from build123d import *

# Parameters (mm, degrees)
EXTRUDE_1_DEPTH       = 244
EXTRUDE_3_DEPTH       = 244
PATTERN_CURVE_1_DEPTH = 244
SKETCH_3_R            = 2.25
CUT_EXTRUDE_1_DEPTH   = 6
SKETCH_4_R            = 1.6
SKETCH_4_R_2          = 1.15
CUT_EXTRUDE_2_DEPTH   = 6


# Read off the part's stored shape, not the designer's step: the pattern curve step
with BuildPart() as part:
    # Sketch 1 → Extrude 1 (new body)
    with BuildSketch(Plane.XY):
        with BuildLine():
            Line((0, 40), (1.528979332, 40))
            ThreePointArc((1.528979332, 40), (2.225614441, 39.717425624), (2.528547087, 39.029399052))
            Line((2.528547087, 39.029399052), (3.5, 6))
            Line((3.5, 6), (118.5, 6))
            Line((118.5, 6), (119.471452913, 39.029399052))
            ThreePointArc((119.471452913, 39.029399052), (119.774385559, 39.717425624), (120.471020668, 40))
            Line((120.471020668, 40), (122, 40))
            Line((122, 40), (122, 0))
            Line((122, 0), (0, 0))
            Line((0, 0), (0, 40))
        make_face()
    extrude(amount=EXTRUDE_1_DEPTH)

    # Sketch 2 → Extrude 3 (add)
    with BuildSketch(Plane.XY.offset(244)):
        with BuildLine():
            Line((10.5, 39.5), (9.25, 6))
            Line((9.25, 6), (12.75, 6))
            Line((12.75, 6), (11.5, 39.5))
            ThreePointArc((11.5, 39.5), (11, 40), (10.5, 39.5))
        make_face()
    extrude(amount=-EXTRUDE_3_DEPTH)

    # Pattern Curve 1 outline → Pattern Curve 1 (add)
    with BuildSketch(Plane.XY):
        with BuildLine():
            ThreePointArc((21.5, 39.5), (21, 40), (20.5, 39.5))
            Line((20.5, 39.5), (19.25, 6))
            Line((19.25, 6), (22.75, 6))
            Line((22.75, 6), (21.5, 39.5))
        make_face()
        with BuildLine():
            Line((110.5, 39.5), (109.25, 6))
            Line((109.25, 6), (112.75, 6))
            Line((112.75, 6), (111.5, 39.5))
            ThreePointArc((111.5, 39.5), (111, 40), (110.5, 39.5))
        make_face()
        with BuildLine():
            Line((100.5, 39.5), (99.25, 6))
            Line((99.25, 6), (102.75, 6))
            Line((102.75, 6), (101.5, 39.5))
            ThreePointArc((101.5, 39.5), (101, 40), (100.5, 39.5))
        make_face()
        with BuildLine():
            Line((90.5, 39.5), (89.25, 6))
            Line((89.25, 6), (92.75, 6))
            Line((92.75, 6), (91.5, 39.5))
            ThreePointArc((91.5, 39.5), (91, 40), (90.5, 39.5))
        make_face()
        with BuildLine():
            Line((80.5, 39.5), (79.25, 6))
            Line((79.25, 6), (82.75, 6))
            Line((82.75, 6), (81.5, 39.5))
            ThreePointArc((81.5, 39.5), (81, 40), (80.5, 39.5))
        make_face()
        with BuildLine():
            Line((70.5, 39.5), (69.25, 6))
            Line((69.25, 6), (72.75, 6))
            Line((72.75, 6), (71.5, 39.5))
            ThreePointArc((71.5, 39.5), (71, 40), (70.5, 39.5))
        make_face()
        with BuildLine():
            Line((60.5, 39.5), (59.25, 6))
            Line((59.25, 6), (62.75, 6))
            Line((62.75, 6), (61.5, 39.5))
            ThreePointArc((61.5, 39.5), (61, 40), (60.5, 39.5))
        make_face()
        with BuildLine():
            Line((50.5, 39.5), (49.25, 6))
            Line((49.25, 6), (52.75, 6))
            Line((52.75, 6), (51.5, 39.5))
            ThreePointArc((51.5, 39.5), (51, 40), (50.5, 39.5))
        make_face()
        with BuildLine():
            Line((40.5, 39.5), (39.25, 6))
            Line((39.25, 6), (42.75, 6))
            Line((42.75, 6), (41.5, 39.5))
            ThreePointArc((41.5, 39.5), (41, 40), (40.5, 39.5))
        make_face()
        with BuildLine():
            Line((30.5, 39.5), (29.25, 6))
            Line((29.25, 6), (32.75, 6))
            Line((32.75, 6), (31.5, 39.5))
            ThreePointArc((31.5, 39.5), (31, 40), (30.5, 39.5))
        make_face()
    extrude(amount=PATTERN_CURVE_1_DEPTH)

    # Sketch 3 → Cut-Extrude 1 (cut)
    with BuildSketch(Plane.XZ):
        with Locations((26, 236)):
            Circle(SKETCH_3_R)
        with Locations((96, 236)):
            Circle(SKETCH_3_R)
        with Locations(Location((96, 8, 0), (0, 0, 180))):
            Circle(SKETCH_3_R)
        with Locations(Location((26, 8, 0), (0, 0, 180))):
            Circle(SKETCH_3_R)
    extrude(amount=-CUT_EXTRUDE_1_DEPTH, mode=Mode.SUBTRACT)

    # Sketch 4 → Cut-Extrude 2 (cut)
    with BuildSketch(Plane(origin=(133.240090243, 0, 310.149074448), x_dir=(-1, 0, 0), z_dir=(0, -1, 0))):
        with Locations((8.990090243, 225.549074448)):
            Circle(SKETCH_4_R)
        with Locations(Location((83.240090243, 178.149074448, 0), (0, 0, 180))):
            Circle(SKETCH_4_R_2)
        with Locations(Location((69.240090243, 163.149074448, 0), (0, 0, 180))):
            Circle(SKETCH_4_R)
        with Locations(Location((61.240090243, 283.149074448, 0), (0, 0, 180))):
            Circle(SKETCH_4_R)
        with Locations(Location((61.240090243, 178.149074448, 0), (0, 0, 180))):
            Circle(SKETCH_4_R)
        with Locations(Location((107.240090243, 178.149074448, 0), (0, 0, 180))):
            Circle(SKETCH_4_R_2)
    extrude(amount=-CUT_EXTRUDE_2_DEPTH, mode=Mode.SUBTRACT)


solid = part.part
Build history of the part. All positions in model axes, mm. A direction names the side the tool comes from. Coordinates: 2 decimals unless noted, no trailing zeros. Use CSV: the item, a comma, the result in double quotes. Start each with the question number.
Q1. 3-axis set-ups, long thin cutter, end or side, ignore diameter. For faces 3 (the flat face through (0, 20, 120)), 4 (the flat face through (46, 6, 120)): which of +Z, -Z, +X, -X, +Y, -Y reach the whole face in a straight line?
Q2. Flat gauge pins, fed straight in: pin 1 Ø3 at (x, z) = (7.5, 122) entering from +Y; pin 2 Ø4 at (x, z) = (96, 236) entering from -Y; pin 3 Ø2 at (x, z) = (50, 132) entering from -Y. Where does each tip first touch, or does it go through?
Q3. Drill centre lines: probe 1 along Z at (x, y) = (26, 4); probe 2 along Z at (x, y) = (96, 2); probe 3 along Z at (x, y) = (72, 1.55). Where is each one in solid material? Low to high.
Q4. Cut at A-A, the plane y = 22.5. State how many separate pieces and enclosed holes the cut face has, then the cut area to 3 significant figures.
Q5. Pull direction Z, two halves, no side cores. Call faces 1 (the cylindrical face through (23.854, 2.958, 7.324)), 2 (the flat face through (92.134, 22.516, 120.292)): released by +Z, released by -Z, zero draft, split by the parting line, or undercut.
Checked values:
1,face 3,"+Z, -Z, -X, +Y, -Y"
1,face 4,"+Z, -Z, +Y"
2,pin 1,"stops at y = 6"
2,pin 2,"passes through"
2,pin 3,"stops at y = 6"
3,probe 1,"z = 0 to 5.75, 10.25 to 130.85, 133.15 to 233.75, 238.25 to 244"
3,probe 2,"z = 0 to 5.75, 10.25 to 233.75, 238.25 to 244"
3,probe 3,"z = 0 to 25.4, 28.6 to 130.4, 133.6 to 244"
4,separate pieces,"13"
4,enclosed holes,"0"
4,area,"7,560 mm²"
5,face 1,"undercut"
5,face 2,"zero draft"
